from build123d import *

# Parameters (mm, degrees)
SKETCH1_W           = 5
SKETCH1_H           = 10
BOSS_EXTRUDE1_DEPTH = 10
SKETCH2_R           = 1.5
CUT_EXTRUDE1_DEPTH  = 16
FILLET1_R           = 4


with BuildPart() as part:
    # Sketch1 → Boss-Extrude1 (new body)
    with BuildSketch(Plane.XY):
        with Locations((2.5, 5)):
            Rectangle(SKETCH1_W, SKETCH1_H)
    extrude(amount=BOSS_EXTRUDE1_DEPTH)

    # Sketch2 → Cut-Extrude1 (cut, through all)
    with BuildSketch(Plane.ZY):
        with Locations((5, 3)):
            Circle(SKETCH2_R)
    extrude(amount=-CUT_EXTRUDE1_DEPTH, mode=Mode.SUBTRACT)

    # Fillet1
    fillet1_edges = [part.edges().sort_by_distance(p)[0] for p in [
        (2.5, 0, 0),
        (2.5, 0, 10),
    ]]
    fillet(fillet1_edges, radius=FILLET1_R)


solid = part.part
The model under review builds one solid part; all positions refer to its coordinate system, in mm. Round coordinates to 2 decimals unless told otherwise and drop trailing zeros. Loops run counter-clockwise (first coordinate to the right, second up) from the corner with the lowest first, then second, coordinate; pieces in that order, holes last. Notation, with made-up numbers: M -29.75,-5 L 25.25,-5 A25 ccw 25.25,8 Z; hole C 39.5,23 d4. An arc over 180 degrees is marked long. Answer as CSV lines item,"result".
1. To check wall thickness, follow L1, parallel to Y at x = 4.25, z = 5; L2, parallel to Y at x = 1.65, z = 3.75; L3, parallel to Z at x = 1.4, y = 1.25. State the ranges of each line that lie inside material, in increasing order. Write a range as [from, to].
Outcome:
L1,"y = [0, 1.5], [4.5, 10]"
L2,"y = [0.01, 2.17], [3.83, 10]"
L3,"z = [1.1, 8.9]"
2. Draft analysis for pull direction Z (two halves, no side actions). For faces 1 (the face through (0, 6, 5)), 2 (the face through (2.46, 1.67, 5.69)), 3 (the face through (2, 7, 10)), state which applies: pulls with the +Z half, pulls with the -Z half, needs draft (parallel to the pull), parting line crosses it, or undercut.
Outcome:
face 1,"needs draft"
face 2,"undercut"
face 3,"pulls with the +Z half"
3. We need section A-A (z = 5). Give the boundary of the cut face in (x, y).
Outcome:
outline,"M 0,0 L 5,0 L 5,1.5 L 0,1.5 Z; M 0,4.5 L 5,4.5 L 5,10 L 0,10 Z"
4. We need section B-B (x = 4.55). Give the boundary of the cut face in (y, z).
Outcome:
outline,"M 0,4 A4 ccw 4,0 L 10,0 L 10,10 L 4,10 A4 ccw 0,6 Z; hole C 3,5 d3"
5. We need section C-C (y = 1.75). Give the boundary of the cut face in (x, z), plus the area to 3 significant figures.
Outcome:
outline,"M 0,0.69 L 5,0.69 L 5,4.17 L 0,4.17 Z; M 0,5.83 L 5,5.83 L 5,9.31 L 0,9.31 Z"
area,"34.8 mm2"
6. We need section D-D (z = 2.25). Give the boundary of the cut face in (x, y).
Outcome:
outline,"M 0,0.4 L 5,0.4 L 5,10 L 0,10 Z"
